For this review, take the finished solid that the model builds, in its own axes (mm). Face numbers are marked on the shaded views. A direction names the side the tool comes from. Give positions to 0.01 mm unless a question says otherwise; leave off trailing zeros. Write each loop counter-clockwise with the first axis right and the second up, starting at its lowest first coordinate (ties: lowest second). Pieces come first, ordered by that corner, then holes.
Q1. We need section D-D (z = 6). Give the number of separate pieces and of enclosed holes in the cut face, then the cut area to 3 significant figures.
Q2. We need section C-C (y = 14.5). Write out the cut boundary in (x, z).
Q3. Insertion check: P1, Ø1.9, axis at x = 21.5, z = 4.5, coming from the -Y side (3 decimals); P2, Ø3.5, axis at x = -19.5, z = 2.5, coming from the +Y side; P3, Ø2, axis at x = 23.5, z = 6, coming from the +Y side (3 decimals). Each pin has a flat end and moves straight along its axis. Give the tip position at first contact, or say it passes through.
Q4. Machinability: for the marked faces 4, 5 and 6, which of the approach directions +Z, -Z, +X, -X, +Y, -Y give a long, thin tool a straight path to every point of the face, cutting with its end or side? Answer none if there is none.
Q5. For line 1 (Y direction, x = 23, z = 6) (3 decimals); line 2 (Y direction, x = -21, z = 2.25) (3 decimals); line 3 (X direction, y = -14, z = 4), list the stretches that pass through material, from the lowest coordinate up.
Q6. We need section B-B (x = 0). Write out the cut boundary in (y, z) (3 decimals), then the cut area to 3 significant figures.
Q7. Mouldability with a two-part tool opening along X and no side actions: class the marked faces 1, 2 and 3 as released by +X, released by -X, zero draft, split by the parting line, or undercut.
Q8. We need section A-A (y = 0). Write out the cut boundary in (x, z).
```python
from build123d import *

# Parameters (mm, degrees)
F0_W     = 2.54
F0_H     = 8.7372876405
F0_H_2   = 8.89
F1_DEPTH = 6.9977
F2_R     = 11.176
F3_DEPTH = 6.9977


with BuildPart() as f1:
    # F0 (on Top) → F1 (new body)
    with BuildSketch(Plane.XY):
        Polygon((-11.6335226281, 5.2501477372), (-10.3635226281, 7.4498522628), (-14.0807527651, 9.595996083), (-15.3507527651, 7.3962915574), align=None)
        Polygon((-14.6646968374, 0), (-11.6335226281, 5.2501477372), (-15.3507527651, 7.3962915574), (-17.1428502621, 4.2922876405), (-20.7270452561, 4.2922876405), (-20.7270452561, -4.445), (-17.231018784, -4.445), (-15.4830055479, -7.4726477372), (-11.6335226281, -5.2501477372), align=None)
        Polygon((-15.3507527651, 7.3962915574), (-14.0807527651, 9.595996083), (-12.3768237899, 12.5472876405), (-14.124837026, 15.5749353777), (-14.2130055479, 15.7276477372), (-15.394837026, 17.7746399033), (-17.1428502621, 20.8022876405), (-26.6749032064, 20.8022876405), (-31.4409296786, 12.5472876405), (-26.6749032064, 4.2922876405), (-23.2670452561, 4.2922876405), (-20.7270452561, 4.2922876405), (-17.1428502621, 4.2922876405), align=None)
        Polygon((-18.7559669142, 18.0082876405), (-15.6030570942, 12.5472876405), (-18.7559669142, 7.0862876405), (-25.0617865543, 7.0862876405), (-28.2146963743, 12.5472876405), (-25.0617865543, 18.0082876405), align=None, mode=Mode.SUBTRACT)
        Polygon((14.2130055479, 9.6723522628), (10.3635226281, 7.4498522628), (11.6335226281, 5.2501477372), (15.4830055479, 7.4726477372), align=None)
        Polygon((-10.3635226281, -7.4498522628), (-11.6335226281, -5.2501477372), (-15.4830055479, -7.4726477372), (-14.2130055479, -9.6723522628), align=None)
        Polygon((-14.2130055479, 15.7276477372), (-14.124837026, 15.5749353777), (-6.4258711864, 20.0199353777), (-7.6958711864, 22.2196399033), (-15.394837026, 17.7746399033), align=None)
        Polygon((15.4830055479, 7.4726477372), (11.6335226281, 5.2501477372), (14.6646968374, 0), (11.6335226281, -5.2501477372), (15.4830055479, -7.4726477372), (17.231018784, -4.445), (20.7270452561, -4.445), (20.7270452561, 4.445), (17.231018784, 4.445), align=None)
        Polygon((12.4649923118, 12.7), (14.2130055479, 9.6723522628), (15.4830055479, 7.4726477372), (17.231018784, 4.445), (20.7270452561, 4.445), (23.2670452561, 4.445), (26.7630717283, 4.445), (31.5290982004, 12.7), (26.7630717283, 20.955), (17.231018784, 20.955), (15.4830055479, 17.9273522628), (14.2130055479, 15.7276477372), align=None)
        Polygon((25.1499550762, 7.239), (18.8441354361, 7.239), (15.691225616, 12.7), (18.8441354361, 18.161), (25.1499550762, 18.161), (28.3028648962, 12.7), align=None, mode=Mode.SUBTRACT)
        Polygon((-14.2130055479, -9.6723522628), (-15.4830055479, -7.4726477372), (-17.231018784, -4.445), (-20.7270452561, -4.445), (-23.2670452561, -4.445), (-26.7630717283, -4.445), (-31.5290982004, -12.7), (-26.7630717283, -20.955), (-17.231018784, -20.955), (-15.4830055479, -17.9273522628), (-14.2130055479, -15.7276477372), (-12.4649923118, -12.7), align=None)
        Polygon((-25.1499550762, -7.239), (-18.8441354361, -7.239), (-15.691225616, -12.7), (-18.8441354361, -18.161), (-25.1499550762, -18.161), (-28.3028648962, -12.7), align=None, mode=Mode.SUBTRACT)
        with Locations((-21.9970452561, -0.0763561798)):
            Rectangle(F0_W, F0_H)
        Polygon((-7.6958711864, 22.2196399033), (-6.4258711864, 20.0199353777), (-4.6778579503, 16.9922876405), (-1.27, 16.9922876405), (1.27, 16.9922876405), (4.854194994, 16.9922876405), (6.6462924911, 20.0962915574), (7.9162924911, 22.295996083), (9.6202214662, 25.2472876405), (4.854194994, 33.5022876405), (-4.6778579503, 33.5022876405), (-9.4438844224, 25.2472876405), align=None)
        Polygon((6.3924737908, 25.3854774003), (3.3599969989, 19.8566940043), (-2.94430827, 19.7185042444), (-6.216136747, 25.1090978806), (-3.1836599552, 30.6378812766), (3.1206453137, 30.7760710365), align=None, mode=Mode.SUBTRACT)
        Polygon((15.4830055479, -7.4726477372), (11.6335226281, -5.2501477372), (10.3635226281, -7.4498522628), (14.2130055479, -9.6723522628), align=None)
        Polygon((6.6462924911, 20.0962915574), (14.2130055479, 15.7276477372), (15.4830055479, 17.9273522628), (7.9162924911, 22.295996083), align=None)
        Polygon((17.231018784, -4.445), (15.4830055479, -7.4726477372), (14.2130055479, -9.6723522628), (12.4649923118, -12.7), (14.2130055479, -15.7276477372), (15.4830055479, -17.9273522628), (17.231018784, -20.955), (26.7630717283, -20.955), (31.5290982004, -12.7), (26.7630717283, -4.445), (23.2670452561, -4.445), (20.7270452561, -4.445), align=None)
        Polygon((18.8441354361, -18.161), (15.691225616, -12.7), (18.8441354361, -7.239), (25.1499550762, -7.239), (28.3028648962, -12.7), (25.1499550762, -18.161), align=None, mode=Mode.SUBTRACT)
        with Locations((21.9970452561, 0)):
            Rectangle(F0_W, F0_H_2)
        Polygon((-6.5140397082, -20.1726477372), (-14.2130055479, -15.7276477372), (-15.4830055479, -17.9273522628), (-7.7840397082, -22.3723522628), align=None)
        Polygon((-4.7660264722, -17.145), (-6.5140397082, -20.1726477372), (-7.7840397082, -22.3723522628), (-9.5320529443, -25.4), (-4.7660264722, -33.655), (4.7660264722, -33.655), (9.5320529443, -25.4), (7.7840397082, -22.3723522628), (6.5140397082, -20.1726477372), (4.7660264722, -17.145), (1.27, -17.145), (-1.27, -17.145), align=None)
        Polygon((-6.3058196401, -25.4), (-3.15290982, -19.939), (3.15290982, -19.939), (6.3058196401, -25.4), (3.15290982, -30.861), (-3.15290982, -30.861), align=None, mode=Mode.SUBTRACT)
        Polygon((15.4830055479, -17.9273522628), (14.2130055479, -15.7276477372), (6.5140397082, -20.1726477372), (7.7840397082, -22.3723522628), align=None)
    extrude(amount=F1_DEPTH)

    # F2 (on Top) → F3 (join)
    with BuildSketch(Plane.XY):
        Polygon((7.6989658396, 13.335), (-7.6989658396, 13.335), (-15.3979316793, 0), (-7.6989658396, -13.335), (7.6989658396, -13.335), (15.3979316793, 0), align=None)
        Circle(F2_R, mode=Mode.SUBTRACT)
    extrude(amount=F3_DEPTH)


solid = f1.part
```
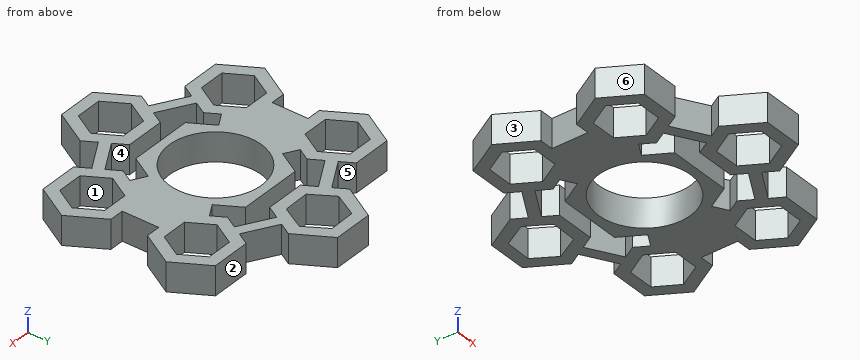
Computed:
1. separate pieces: 1
1. enclosed holes: 9
1. area: 1,350 mm2
2. outline: (-30.31, 0) - (-27.09, 0) - (-27.09, 7) - (-30.31, 7) - close; (-16.73, 0) - (-13.5, 0) - (-13.5, 7) - (-16.73, 7) - close; (13.5, 0) - (16.73, 0) - (16.73, 7) - (13.5, 7) - close; (27.26, 0) - (30.49, 0) - (30.49, 7) - (27.26, 7) - close
3. P1: stops at y = -20.955
3. P2: stops at y = 20.8
3. P3: stops at y = 20.955
4. face 4: +Z, -Z
4. face 5: +Z, -Z, +Y
4. face 6: +Z, -Z, -X, -Y
5. line 1: y = -20.955 to -18.161, -7.239 to 7.239, 18.161 to 20.955
5. line 2: y = -20.955 to -18.161, -7.239 to 7.086, 18.008 to 20.802
5. line 3: x = -30.78 to -27.55, -16.44 to -13.22, 13.22 to 16.44, 27.55 to 30.78
6. outline: (-33.655, 0) - (-30.861, 0) - (-30.861, 6.998) - (-33.655, 6.998) - close; (-19.939, 0) - (-17.145, 0) - (-17.145, 6.998) - (-19.939, 6.998) - close; (-13.335, 0) - (-11.176, 0) - (-11.176, 6.998) - (-13.335, 6.998) - close; (11.176, 0) - (13.335, 0) - (13.335, 6.998) - (11.176, 6.998) - close; (16.992, 0) - (19.783, 0) - (19.783, 6.998) - (16.992, 6.998) - close; (30.708, 0) - (33.502, 0) - (33.502, 6.998) - (30.708, 6.998) - close
6. area: 108 mm2
7. face 1: undercut
7. face 2: zero draft
7. face 3: released by -X
8. outline: (-23.27, 0) - (-11.18, 0) - (-11.18, 7) - (-23.27, 7) - close; (11.18, 0) - (23.27, 0) - (23.27, 7) - (11.18, 7) - close
